from build123d import *

# Parameters (mm, degrees)
SKETCH10_R                = 1
BOSS_EXTRUDE5_DEPTH       = 7.5
CUT_EXTRUDE1_DEPTH        = 4
FILLET1_R                 = 10
CUT_EXTRUDE6_START        = -11
CUT_EXTRUDE6_DEPTH        = 10
CUT_EXTRUDE7_DEPTH        = 2
BOSS_EXTRUDE11_DEPTH      = 9
BOSS_EXTRUDE13_DEPTH      = 64
BOSS_EXTRUDE13_DEPTH_BACK = 3
SKETCH30_W                = 2
SKETCH30_H                = 15
BOSS_EXTRUDE14_DEPTH      = 14
BOSS_EXTRUDE14_DEPTH_BACK = 4
SKETCH31_W                = 1.5
SKETCH31_H                = 29.5
SKETCH31_W_2              = 0.5
SKETCH31_H_2              = 3.0862264
CUT_EXTRUDE9_DEPTH        = 9
FILLET2_R                 = 8
FILLET3_R                 = 10
BOSS_EXTRUDE15_DEPTH      = 2
BOSS_EXTRUDE16_START      = 2
BOSS_EXTRUDE16_DEPTH      = 2
CUT_EXTRUDE10_DEPTH       = 28


with BuildPart() as part:
    # Sketch10 → Boss-Extrude5 (new, symmetric)
    with BuildSketch(Plane.XY):
        Polygon((27.048887868, 48.656944563), (33.959433176, 37.989988632), (36.993816658, 26.682834617), (12.788755024, 23.658848526), (10.279677841, 36.875809012), (12.321789019, 48.656944563), align=None)
        with Locations((17.890076876, 43.12952492)):
            Circle(SKETCH10_R, mode=Mode.SUBTRACT)
        with Locations((23.882298789, 39.668364252)):
            Circle(SKETCH10_R, mode=Mode.SUBTRACT)
    extrude(amount=BOSS_EXTRUDE5_DEPTH, both=True)

    # Sketch11 → Cut-Extrude1 (cut)
    with BuildSketch(Plane.XY.offset(7.5)):
        with BuildLine():
            Line((17.825431655, 32.423947427), (9.123881611, 30.207909529))
            Line((9.123881611, 30.207909529), (6.594316119, 53.15991455))
            Line((6.594316119, 53.15991455), (34.693470887, 60.271659822))
            Line((34.693470887, 60.271659822), (37.752907488, 30.846026516))
            add(Edge.make_bspline(
                [(37.752907488, 30.846026516), (30.679137573, 30.15507536), (19.269012528, 26.734198276), (17.825431655, 32.423947427)],
                knots=[0, 0, 0, 0, 1, 1, 1, 1], degree=3))
        make_face()
    extrude(amount=-CUT_EXTRUDE1_DEPTH, mode=Mode.SUBTRACT)

    # Fillet1
    fillet1_edges = [part.edges().sort_by_distance(p)[0] for p in [
        (27.048887868, 48.656944563, -2),
    ]]
    fillet(fillet1_edges, radius=FILLET1_R)

    # Sketch11<2> → Cut-Extrude6 (cut)
    with BuildSketch(Plane.XY.offset(7.5).offset(CUT_EXTRUDE6_START)):
        with BuildLine():
            Line((17.825431655, 32.423947427), (9.123881611, 30.207909529))
            Line((9.123881611, 30.207909529), (6.594316119, 53.15991455))
            Line((6.594316119, 53.15991455), (34.693470887, 60.271659822))
            Line((34.693470887, 60.271659822), (37.752907488, 30.846026516))
            add(Edge.make_bspline(
                [(37.752907488, 30.846026516), (30.679137573, 30.15507536), (19.269012528, 26.734198276), (17.825431655, 32.423947427)],
                knots=[0, 0, 0, 0, 1, 1, 1, 1], degree=3))
        make_face()
    extrude(amount=-CUT_EXTRUDE6_DEPTH, mode=Mode.SUBTRACT)

    # Sketch16 → Cut-Extrude7 (cut, symmetric)
    with BuildSketch(Plane.XY):
        Polygon((10.074284509, 54.36084815), (34.418624568, 54.36084815), (34.418624568, 36.664364271), (10.074284509, 40.645108775), align=None)
    extrude(amount=CUT_EXTRUDE7_DEPTH, both=True, mode=Mode.SUBTRACT)

    # Sketch26 → Boss-Extrude11 (add)
    with BuildSketch(Plane(origin=(41.188168375, 11.053240949, 0), x_dir=(0, 0, -1), z_dir=(0.9658266565657433, 0.2591888683316433, 0))):
        Polygon((2, 27.88983665), (2, 26.535626274), (-2, 26.535626274), (-2, 27.88983665), (-3.5, 27.88983665), (-3.5, 20.267140373), (-7.5, 20.267140373), (-7.5, 16.182607471), (7.5, 16.182607471), (7.5, 20.267140372), (3.5, 20.267140373), (3.5, 27.88983665), align=None)
    extrude(amount=BOSS_EXTRUDE11_DEPTH)

    # Sketch30 → Boss-Extrude13 (add, two sides: drawn at the far end of the back side and taken through both)
    with BuildSketch(Plane(origin=(-4.194351717, 15.629593668, 0), x_dir=(0.9658266565657433, 0.25918886833164334, 0), z_dir=(0.25918886833164334, -0.9658266565657433, 0)).offset(-BOSS_EXTRUDE13_DEPTH_BACK)):
        with Locations((27.645507965, 0)):
            Rectangle(SKETCH30_W, SKETCH30_H)
        with Locations((25.645507965, 0)):
            Rectangle(SKETCH30_W, SKETCH30_H)
    extrude(amount=BOSS_EXTRUDE13_DEPTH + BOSS_EXTRUDE13_DEPTH_BACK)

    # Sketch31 → Boss-Extrude14 (add, two sides: drawn at the far end of the back side and taken through both)
    with BuildSketch(Plane(origin=(27.666595183, 7.424596792, 0), x_dir=(0, 0, -1), z_dir=(0.9658266565657432, 0.2591888683316434, 0)).offset(-BOSS_EXTRUDE14_DEPTH_BACK)):
        with Locations((-6.75, -32.567392529)):
            Rectangle(SKETCH31_W, SKETCH31_H)
        with Locations((-7.75, -32.567392529)):
            Rectangle(SKETCH31_W_2, SKETCH31_H)
        with Locations((6.75, -32.567392529)):
            Rectangle(SKETCH31_W, SKETCH31_H)
        with Locations((7.75, -32.567392529)):
            Rectangle(SKETCH31_W_2, SKETCH31_H)
        Polygon((-3, -47.317392529), (-6, -47.317392529), (-7.5, -47.317392529), (-7.5, -47.817392529), (-3, -47.817392529), align=None)
        Polygon((7.5, -47.817392529), (3, -47.817392529), (3, -49.317392529), (8, -49.317392529), (8, -47.317392529), (7.5, -47.317392529), align=None)
        Polygon((3, -47.317392529), (3, -47.817392529), (7.5, -47.817392529), (7.5, -47.317392529), (6, -47.317392529), align=None)
        Polygon((-7.5, -47.817392529), (-7.5, -47.317392529), (-8, -47.317392529), (-8, -49.317392529), (-3, -49.317392529), (-3, -47.817392529), align=None)
        Polygon((-7.5, -17.817392529), (-6, -17.817392529), (-3.25, -17.817392529), (-3.25, -14.731166129), (-7.5, -14.731166129), align=None)
        Polygon((3.25, -17.817392529), (6, -17.817392529), (7.5, -17.817392529), (7.5, -14.731166129), (3.25, -14.731166129), align=None)
        with Locations((7.75, -16.274279329)):
            Rectangle(SKETCH31_W_2, SKETCH31_H_2)
        with Locations((-7.75, -16.274279329)):
            Rectangle(SKETCH31_W_2, SKETCH31_H_2)
    extrude(amount=BOSS_EXTRUDE14_DEPTH + BOSS_EXTRUDE14_DEPTH_BACK)

    # Sketch32 → Cut-Extrude9 (cut)
    with BuildSketch(Plane(origin=(49.880608284, 13.385940764, 0), x_dir=(0, 0, -1), z_dir=(0.9658266565657431, 0.25918886833164445, 0))):
        Polygon((3.5, 27.88983665), (2, 27.88983665), (2, 26.535626274), (-2, 26.535626274), (-2, 27.88983665), (-3.5, 27.88983665), (-3.5, 20.267140373), (-7.5, 20.267140373), (-7.5, 16.182607471), (7.5, 16.182607471), (7.5, 20.267140372), (3.5, 20.267140373), align=None)
    extrude(amount=-CUT_EXTRUDE9_DEPTH, mode=Mode.SUBTRACT)

    # Fillet2
    fillet2_edges = [part.edges().sort_by_distance(p)[0] for p in [
        (12.321789019, 48.656944563, 2.75),
        (12.321789019, 48.656944563, -2.75),
    ]]
    fillet(fillet2_edges, radius=FILLET2_R)

    # Fillet3
    fillet3_edges = [part.edges().sort_by_distance(p)[0] for p in [
        (17.825431655, 32.423947427, 5.5),
        (17.825431655, 32.423947427, -5.5),
    ]]
    fillet(fillet3_edges, radius=FILLET3_R)

    # Sketch33 → Boss-Extrude15 (add)
    with BuildSketch(Plane(origin=(0, 0, -7.5), x_dir=(-1, 0, 0), z_dir=(0, 0, -1))):
        with BuildLine():
            Line((-11.433819556, 30.796185182), (-12.326379112, 31.023494775))
            ThreePointArc((-12.326379112, 31.023494775), (-16.080268918, 31.249787506), (-19.652288318, 30.073533078))
            add(Edge.make_bspline(
                [(-19.652288318, 30.073533078), (-23.094178016, 28.160579122), (-30.349802092, 29.858629099), (-35.935151197, 30.627785373)],
                knots=[0.191604014, 0.191604014, 0.191604014, 0.191604014, 0.918085752, 0.918085752, 0.918085752, 0.918085752], degree=3))
            Line((-35.935151197, 30.627785373), (-36.993816658, 26.682834617))
            Line((-36.993816658, 26.682834617), (-22.968678464, 24.93064644))
            Line((-22.968678464, 24.93064644), (-31.484749461, -6.803156137))
            Line((-31.484749461, -6.803156137), (-27.621442835, -7.839911611))
            Line((-27.621442835, -7.839911611), (-18.961496124, 24.430021246))
            Line((-18.961496124, 24.430021246), (-12.788755024, 23.658848526))
            Line((-12.788755024, 23.658848526), (-11.433819556, 30.796185182))
        make_face()
    extrude(amount=BOSS_EXTRUDE15_DEPTH)

    # Sketch34 → Boss-Extrude16 (add)
    with BuildSketch(Plane.XY.offset(7.5).offset(BOSS_EXTRUDE16_START)):
        with BuildLine():
            Line((12.326379112, 31.023494775), (11.433819556, 30.796185182))
            Line((11.433819556, 30.796185182), (12.788755024, 23.658848526))
            Line((12.788755024, 23.658848526), (22.968678464, 24.93064644))
            Line((22.968678464, 24.93064644), (36.993816658, 26.682834617))
            Line((36.993816658, 26.682834617), (35.935151197, 30.627785373))
            add(Edge.make_bspline(
                [(35.935151197, 30.627785373), (30.349802091, 29.858629099), (23.094178016, 28.160579122), (19.652288318, 30.073533078)],
                knots=[0.191604014, 0.191604014, 0.191604014, 0.191604014, 0.918085752, 0.918085752, 0.918085752, 0.918085752], degree=3))
            ThreePointArc((19.652288318, 30.073533078), (16.080268918, 31.249787506), (12.326379112, 31.023494775))
        make_face()
    extrude(amount=-BOSS_EXTRUDE16_DEPTH)

    # Sketch36 → Cut-Extrude10 (cut)
    with BuildSketch(Plane.XY.offset(9.5)):
        with BuildLine():
            Line((28.735168536, 45.675741107), (43.151621949, 50.021353904))
            Line((43.151621949, 50.021353904), (48.709339966, 19.453904806))
            Line((48.709339966, 19.453904806), (40.633280972, 13.201472036))
            add(Edge.make_bspline(
                [(28.735168536, 45.675741107), (36.204474426, 33.608717883), (15.102513827, 27.616803145), (34.98872361, 13.201472036), (40.633280972, 13.201472036)],
                knots=[0, 0, 0, 0, 0, 1, 1, 1, 1, 1], degree=4))
        make_face()
    extrude(amount=-CUT_EXTRUDE10_DEPTH, mode=Mode.SUBTRACT)


solid = part.part
Read the model definition and answer for the solid it produces. Units are mm, in the model's axes. A direction names the side the tool comes from. Give positions to 0.01 mm unless a question says otherwise; leave off trailing zeros. Loops run counter-clockwise (first coordinate to the right, second up) from the corner with the lowest first, then second, coordinate; pieces in that order, holes last. Notation, with made-up numbers: (-2.75, 55.25) -> (34.25, 55.25) arc R22 cw to (34.25, 87.25) -> close; hole circle Ø3 at (-20, 88). An arc over 180 degrees is marked (long way). Use a Markdown table: item, result.
Q1. Each of these flat-tipped pins is pushed along its axis until it touches: pin 1 (13 mm diameter, centred on x = 44, y = -17, fed in from -Z); pin 2 (1.6 mm diameter, centred on x = 17.89, y = 43.13, fed in from -Z); pin 3 (6.5 mm diameter, centred on x = 48, y = -17.5, fed in from +Z); pin 4 (5.5 mm diameter, centred on x = 21, y = 43.5, fed in from -Z). Where does it stop, or does it pass through?
Solved:
| item | result |
|---|---|
| pin 1 | stops at z = -8 |
| pin 2 | passes through |
| pin 3 | stops at z = 8 |
| pin 4 | stops at z = -3.5 |
Q2. A tool of negligible diameter and unlimited length cuts with its end or side. For faces 1 (the face through (38.951, -7.995, 4.644)), 2 (the face through (46.597, -36.487, 4.479)), 3 (the face through (38.2, -5, -5.7)), 4 (the face through (22, 44, 2)), 5 (the face through (17.673, 42.153, 2.74)), from which of +Z, -Z, +X, -X, +Y, -Y can it reach the whole face along a straight path? Write none if from no direction.
Solved:
| item | result |
|---|---|
| face 1 | +X |
| face 2 | none |
| face 3 | +Z, -Z, +Y |
| face 4 | +X, +Y |
| face 5 | +Z, -Z |
Q3. Section A-A, the plane x = 47 is taken. Determine the outline of the cut face in (y, z).
Solved:
| item | result |
|---|---|
| outline | (-38.45, -8) -> (-10.6, -8) -> (-10.6, -6) -> (-36.38, -6) -> (-36.38, -3) -> (-38.45, -3) -> close; (-38.45, 3) -> (-36.38, 3) -> (-36.38, 6) -> (-10.6, 6) -> (-10.6, 8) -> (-38.45, 8) -> close |
Q4. Section C-C, the plane x = 18 is taken. Count the separate pieces of the cut face and the enclosed holes in it, then the cut area to 3 significant figures.
Solved:
| item | result |
|---|---|
| separate pieces | 3 |
| enclosed holes | 0 |
| area | 205 mm^2 |
Q5. Find the intervals of material crossed by line 1 along Z through (x, y) = (46, -21.5); line 2 along Z through (x, y) = (23.5, 14.5); line 3 along Z through (x, y) = (18.5, 41.5), in increasing order.
Solved:
| item | result |
|---|---|
| line 1 | z = -8 to -6, 6 to 8 |
| line 2 | z = -9.5 to 7.5 |
| line 3 | z = -3.5 to -2, 2 to 3.5 |
Q6. Section B-B, the plane y = -12 is taken. Determine the outline of the cut face in (x, z), then the cut area to 3 significant figures.
Solved:
| item | result |
|---|---|
| outline | (28.74, -8) -> (47.37, -8) -> (47.37, -6) -> (32.88, -6) -> (32.88, 6) -> (47.37, 6) -> (47.37, 8) -> (28.74, 8) -> close |
| area | 124 mm^2 |
Q7. Section D-D, the plane y = 18 is taken. Determine the outline of the cut face in (x, z), then the cut area to 3 significant figures.
Solved:
| item | result |
|---|---|
| outline | (20.69, -9.5) -> (24.83, -9.5) -> (24.83, 7.5) -> (20.69, 7.5) -> close |
| area | 70.4 mm^2 |
Q8. Determine the mould class of faces 6 (the face through (20, 38, 3.5)), 7 (the face through (39, -6, -3.25)), 8 (the face through (22, 43, -2)), 9 (the face through (23.67, 38.69, 2.74)) for opening direction Z: pulls with the +Z half, pulls with the -Z half, needs draft (parallel to the pull), parting line crosses it, or undercut.
Solved:
| item | result |
|---|---|
| face 6 | pulls with the +Z half |
| face 7 | undercut |
| face 8 | undercut |
| face 9 | needs draft |
